Geometry check sheet. Reference: the model listing, model coordinates, mm. A direction names the side the tool comes from. Coordinates: 2 decimals unless noted, no trailing zeros. Write each loop counter-clockwise with the first axis right and the second up, starting at its lowest first coordinate (ties: lowest second). Pieces come first, ordered by that corner, then holes. Notation, with made-up numbers: (9.25, 55.25) -> (68.25, 55.25) arc R10 cw to (68.25, 69.25) -> close; hole circle Ø8 at (-29, -30). An arc over 180 degrees is marked (long way). One line per question, with ' | ' between items.
```python
from build123d import *

# Parameters (mm, degrees)
SKETCH_1_R          = 2.5
EXTRUDE_1_DEPTH     = 10
SKETCH_3_R          = 1.6
CUT_EXTRUDE_1_DEPTH = 11.955148971


with BuildPart() as part:
    # 草图1 → 凸台-拉伸1 (new body)
    with BuildSketch(Plane.XY):
        Circle(SKETCH_1_R)
    extrude(amount=EXTRUDE_1_DEPTH)

    # 草图2 → 旋转1 (revolve)
    with BuildSketch(Plane(origin=(0, 0, 0), x_dir=(1, 0, 0), z_dir=(0, 1, 0))):
        with BuildLine():
            Line((0, -8), (-2.048968216, -8))
            ThreePointArc((-2.048968216, -8), (-3.117957315, -6.124512969), (-2.735029198, -4))
            Line((-2.735029198, -4), (0, -4))
            Line((0, -4), (0, -8))
        make_face()
    revolve(axis=Axis((0, 0, 8), (0, 0, -1)))

    # 草图3 → 切除-拉伸1 (cut, through all)
    with BuildSketch(Plane.XY.offset(10)):
        Circle(SKETCH_3_R)
    extrude(amount=-CUT_EXTRUDE_1_DEPTH, mode=Mode.SUBTRACT)


solid = part.part
```
(1) Cross-section at A-A (x = 0). Record the cut outline in (y, z), plus the area to 3 significant figures.
Answers below:
outline: (-2.74, 4) -> (-2.5, 4) -> (-2.5, 0) -> (-1.6, 0) -> (-1.6, 10) -> (-2.5, 10) -> (-2.5, 7.53) arc R3.16 ccw to start; (1.6, 0) -> (2.5, 0) -> (2.5, 4) -> (2.74, 4) arc R3.16 ccw to (2.5, 7.53) -> (2.5, 10) -> (1.6, 10) -> close | area: 21.4 mm²
(2) Cross-section at C-C (z = 2). Record the cut outline in (x, y).
Answers below:
outline: circle Ø5 at (0, 0); hole circle Ø3.2 at (0, 0)
(3) Cross-section at D-D (y = 1.75). Record the cut outline in (x, z), plus the area to 3 significant figures.
Answers below:
outline: (-2.1, 4) -> (-1.79, 4) -> (-1.79, 0) -> (1.79, 0) -> (1.79, 4) -> (2.1, 4) arc R2.64 ccw to (1.79, 7.53) -> (1.79, 10) -> (-1.79, 10) -> (-1.79, 7.53) arc R2.64 ccw to start | area: 40.1 mm²
(4) Material ranges on line 1 (Y direction, x = 0, z = 4.5); line 2 (Y direction, x = 0.25, z = 7.75); line 3 (X direction, y = 1.25, z = 1), recorded low to high.
Answers below:
line 1: y = -2.97 to -1.6, 1.6 to 2.97 | line 2: y = -2.49 to -1.58, 1.58 to 2.49 | line 3: x = -2.17 to -1, 1 to 2.17
(5) Tool access check on faces 1 (the face through (0, -2, 10)), 2 (the face through (-0.54, -2.44, 8.75)). Record the directions out of +Z, -Z, +X, -X, +Y, -Y that give a thin tool (end or side, any length) a straight path to the whole face; none if there is none.
Answers below:
face 1: +Z, +X, -X, +Y, -Y | face 2: +Z
(6) Depth check by flat-ended pin: P1, Ø1.5, axis at x = -1, y = 2, coming from the -Z side; P2, Ø3, axis at y = -2, z = 3.5, coming from the -X side; P3, Ø1, axis at y = 1, z = 1.5, coming from the +X side. Enter the tip coordinate at first touch or a pass-through.
Answers below:
P1: stops at z = 0 | P2: stops at x = -2.84 | P3: stops at x = 2.45
(7) Draft check along X on faces 3 (the face through (-0.54, -2.44, 1.97)), 4 (the face through (-1.27, -0.97, 5.07)), 5 (the face through (0, -2, 0)). Enter one of: pulls with the +X half, pulls with the -X half, needs draft (parallel to the pull), parting line crosses it, or undercut.
Answers below:
face 3: parting line crosses it | face 4: undercut | face 5: needs draft
